Could you check a few things on this model? Use its own coordinates, in mm. Face numbers are marked on the shaded views. A direction names the side the tool comes from. Coordinates: 2 decimals unless noted, no trailing zeros. Write each loop counter-clockwise with the first axis right and the second up, starting at its lowest first coordinate (ties: lowest second). Pieces come first, ordered by that corner, then holes. Notation, with made-up numbers: M 37.5,-26 L 65.5,-26 A13 ccw 65.5,-17 Z; hole C 76.5,78.25 d3. An arc over 180 degrees is marked long. Answer as CSV lines item,"result". Start each with the question number.
Item 1: Suppose I cut it at A-A, the plane z = 105. Write out the boundary of the cut face in (x, y), and give its area (3 significant figures).
Item 2: We'd pull the mould along X, two halves only. Please class the marked faces 3, 4 and 5: +X half, -X half, draft (parallel to the pull), parting line (faces both ways), or undercut.
Item 3: Suppose I cut it at D-D, the plane x = 0. Write out the boundary of the cut face in (y, z).
Item 4: On a 3-axis mill with a long thin cutter (end or side, diameter ignored), from which of +Z, -Z, +X, -X, +Y, -Y can I reach the whole of each face in a straight line? I mean the marked faces 1 and 2. Say none if no direction works.
Item 5: I'm going to push flat-ended pins straight in: P1, Ø16, axis at y = 0, z = 105, coming from the -X side; P2, Ø3, axis at x = 0, y = 0, coming from the -Z side; P3, Ø4, axis at x = 0.5, y = -8.5, coming from the +Z side. Where does each tip first touch, or does it pass through?
Item 6: Suppose I cut it at B-B, the plane y = 0. Write out the boundary of the cut face in (x, z).
Item 7: Suppose I cut it at C-C, the plane x = 14.5. Write out the boundary of the cut face in (y, z), and give its area (3 significant figures).
Item 8: If I drill on line 1 along Y through (x, z) = (0, 5); line 2 along Z through (x, y) = (-12.5, 0); line 3 along X through (y, z) = (-4, 100), over which ranges is the centre line in solid material (lowest first)? Write a range as [from, to].
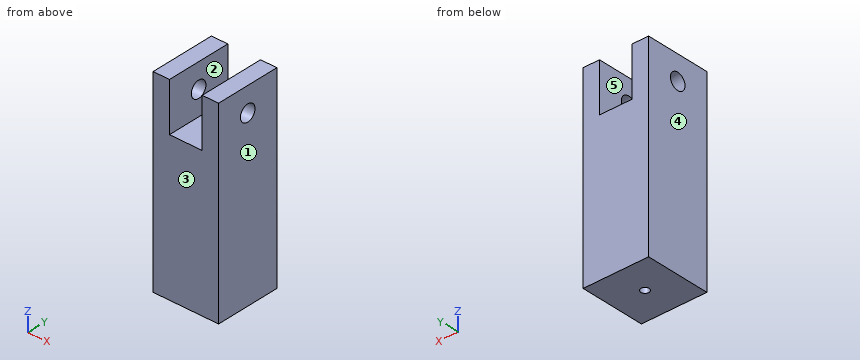
```python
from build123d import *

# Parameters (mm, degrees)
SKICA1_W                 = 40
SKICA1_H                 = 40
P_IDAT_VYSUNUT_M1_DEPTH  = 90
SKICA3_W                 = 10
SKICA3_H                 = 40
P_IDAT_VYSUNUT_M2_DEPTH  = 30
SKICA4_R                 = 5
ODEBRAT_VYSUNUT_M1_DEPTH = 40
SKICA5_R                 = 2.5
ODEBRAT_VYSUNUT_M2_DEPTH = 10


with BuildPart() as part:
    # Skica1 → Přidat vysunutím1 (new body)
    with BuildSketch(Plane.XY):
        Rectangle(SKICA1_W, SKICA1_H)
    extrude(amount=P_IDAT_VYSUNUT_M1_DEPTH)

    # Skica3 → Přidat vysunutím2 (add)
    with BuildSketch(Plane.XY.offset(90)):
        with Locations((15, 0)):
            Rectangle(SKICA3_W, SKICA3_H)
        with Locations((-15, 0)):
            Rectangle(SKICA3_W, SKICA3_H)
    extrude(amount=P_IDAT_VYSUNUT_M2_DEPTH)

    # Skica4 → Odebrat vysunutím1 (cut)
    with BuildSketch(Plane.ZY.offset(20)):
        with Locations(Location((105, 0, 0), (0, 0, 270))):
            Circle(SKICA4_R)
    extrude(amount=-ODEBRAT_VYSUNUT_M1_DEPTH, mode=Mode.SUBTRACT)

    # Skica5 → Odebrat vysunutím2 (cut)
    with BuildSketch(Plane(origin=(0, 0, 0), x_dir=(-1, 0, 0), z_dir=(0, 0, -1))):
        Circle(SKICA5_R)
    extrude(amount=-ODEBRAT_VYSUNUT_M2_DEPTH, mode=Mode.SUBTRACT)


solid = part.part
```
Ans:
1,outline,"M -20,-20 L -10,-20 L -10,-5 L -20,-5 Z; M -20,5 L -10,5 L -10,20 L -20,20 Z; M 10,-20 L 20,-20 L 20,-5 L 10,-5 Z; M 10,5 L 20,5 L 20,20 L 10,20 Z"
1,area,"600 mm^2"
2,face 3,"draft"
2,face 4,"-X half"
2,face 5,"undercut"
3,outline,"M -20,0 L -2.5,0 L -2.5,10 L 2.5,10 L 2.5,0 L 20,0 L 20,90 L -20,90 Z"
4,face 1,"+Z, -Z, +X, +Y, -Y"
4,face 2,"+Z, +Y, -Y"
5,P1,"stops at x = -20"
5,P2,"stops at z = 10"
5,P3,"stops at z = 90"
6,outline,"M -20,0 L -2.5,0 L -2.5,10 L 2.5,10 L 2.5,0 L 20,0 L 20,100 L 10,100 L 10,90 L -10,90 L -10,100 L -20,100 Z; M -20,110 L -10,110 L -10,120 L -20,120 Z; M 10,110 L 20,110 L 20,120 L 10,120 Z"
7,outline,"M -20,0 L 20,0 L 20,120 L -20,120 Z; hole C 0,105 d10"
7,area,"4,720 mm^2"
8,line 1,"y = [-20, -2.5], [2.5, 20]"
8,line 2,"z = [0, 100], [110, 120]"
8,line 3,"x = [-20, -10], [10, 20]"
